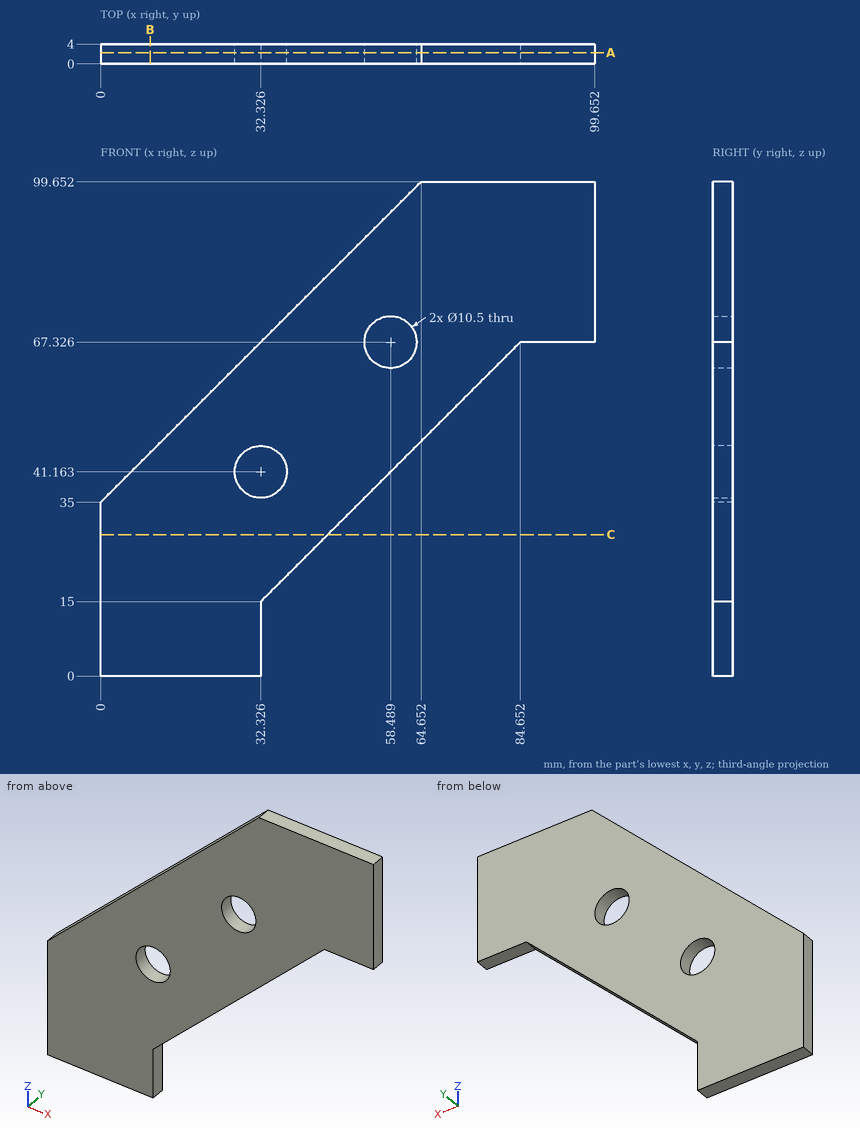
For this review, use the dimensioned drawing (mm, ordinates from the lowest corner) and the shaded views. Coordinates: 2 decimals unless noted, no trailing zeros. Order: outer loops, then holes, each group sorted by start corner. A loop starts at its lowest first (then second) coordinate and runs counter-clockwise, first axis right, second up. Notation, with made-up numbers: (12, 21.5) -> (28, 21.5) arc R20 ccw to (28, 35.5) -> close; hole circle Ø11 at (3.5, 62). An arc over 180 degrees is marked (long way). One line per item, written item: value. Start each with the question number.
Q1. Insertion check: pin 1 Ø1 at (y, z) = (3.5, 74.5) entering from -X; pin 2 Ø2 at (x, y) = (91, 2.5) entering from -Z; pin 3 Ø1 at (x, y) = (79.5, 2.5) entering from -Z. Each pin has a flat end and moves straight along its axis. Give the tip position at first contact, or say it passes through.
Q2. Take a section at B-B, the plane x = 10. State the section outline as (y, z) points, then the cut area to 3 significant figures.
Q3. Take a section at C-C, the plane z = 28.5. State the section outline as (x, y) points.
Q4. For probe 1 along Z at (x, y) = (88.5, 0.75); probe 2 along Z at (x, y) = (33, 2.3) (1 decimal); probe 3 along X at (y, z) = (1.95, 66.5) (1 decimal), list the stretches that pass through material, from the lowest coordinate up.
Q5. Take a section at A-A, the plane y = 2.25. State the section outline as (x, z) points.
Values follow:
1. pin 1: stops at x = 39
1. pin 2: stops at z = 67.33
1. pin 3: stops at z = 61.67
2. outline: (0, 0) -> (4, 0) -> (4, 45) -> (0, 45) -> close
2. area: 180 mm2
3. outline: (0, 0) -> (45.83, 0) -> (45.83, 4) -> (0, 4) -> close
4. probe 1: z = 67.33 to 99.65
4. probe 2: z = 15.7 to 36, 46.4 to 68
4. probe 3: x = 31.5 to 53.3, 63.7 to 83.8
5. outline: (0, 0) -> (32.33, 0) -> (32.33, 15) -> (84.65, 67.33) -> (99.65, 67.33) -> (99.65, 99.65) -> (64.65, 99.65) -> (0, 35) -> close; hole circle Ø10.5 at (32.33, 41.16); hole circle Ø10.5 at (58.49, 67.33)
